Autodesk Inventor part; units mm, degrees
ref_plane "YZ Plane" through (0, 0, 0) normal (1, 0, 0) x (0, 1, 0)
ref_plane "XZ Plane" through (0, 0, 0) normal (0, 1, 0) x (-1, 0, 0)
ref_plane "XY Plane" through (0, 0, 0) normal (0, 0, 1) x (1, 0, 0)
sketch "Sketch1" plane through (0, 0, 0) normal (0, 0, 1) x (1, 0, 0)
  circle A0 centre (0, 0) radius 4
  dimension "Diameter" = 8
extrude "Extrusion1" add sketch "Sketch1" along normal blind 12
sketch "Sketch2" plane through (0, 0, 12) normal (0, 0, 1) x (1, 0, 0)
  circle A0 centre (0, 0) radius 4
  circle A1 centre (0, 0) radius 6.5
  dimension "Head_Diameter" = 13
extrude "Extrusion2" add sketch "Sketch2" along normal blind 8 contours A0 | A1
sketch "Sketch3" plane through (0, 0, 20) normal (0, 0, 1) x (1, 0, 0)
  circle A0 centre (0, 0) radius 6.5
  circle A1 centre (0, 0) radius 3.4641 construction
  line L0 (0, 3.4641) -> (3, 1.7321)
  line L1 (3, -1.7321) -> (3, 1.7321)
  line L2 (0, 3.4641) -> (-3, 1.7321)
  line L3 (-3, -1.7321) -> (-3, 1.7321)
  line L4 (-3, -1.7321) -> (0, -3.4641)
  line L5 (3, -1.7321) -> (0, -3.4641)
  dimension "Hex_Width" = 6
extrude "Extrusion3" cut sketch "Sketch3" against normal blind 4 contours L0 L1 L5 L4 L3 L2
thread "Thread1"
chamfer "Chamfer1" distance 0.8 angle 45 2 edges at (-6.5, 0, 20) (-4, 0, 0)
equation "\"d9\" = ThreadLength"
equation "\"d12\" = Chamfer"
equation "\"ThreadLength\" = 12"
properties part number "SCREW, SOCKET HD, P, 12.9, M8X1.25X12MM" material "Steel, MS"
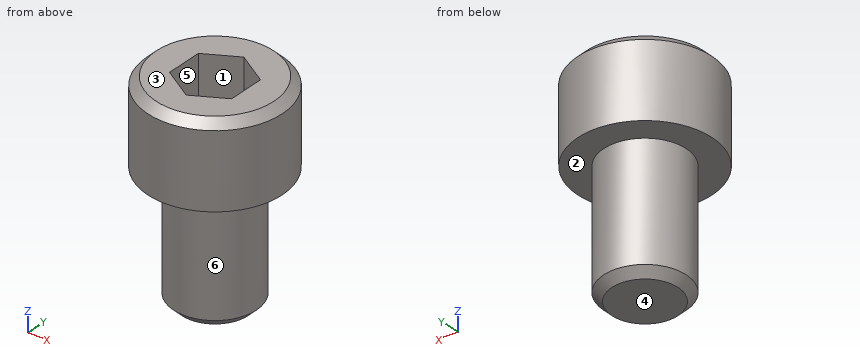
The model under review builds one solid part; all positions refer to its coordinate system, in mm. Face numbers are marked on the shaded views. A direction names the side the tool comes from. Coordinates: 2 decimals unless noted, no trailing zeros. Write each loop counter-clockwise with the first axis right and the second up, starting at its lowest first coordinate (ties: lowest second). Pieces come first, ordered by that corner, then holes. Notation, with made-up numbers: (-39.5, 57.25) - (-1.5, 57.25) arc R20 ccw to (-1.5, 83.25) - close; hole circle Ø6 at (-39, -12). An arc over 180 degrees is marked (long way). Answer as a JSON object with one key per item and string values. Group by question number.
1. To check wall thickness, follow probe 1 along Z at (x, y) = (0.5, -5); probe 2 along X at (y, z) = (-5.5, 17.75); probe 3 along Z at (x, y) = (-2, -0.75). State the ranges of each line that lie inside material, in increasing order.
2. Add section B-B (z = 15). Give the boundary of the cut face in (x, y).
3. Mouldability with a two-part tool opening along X and no side actions: class the marked faces 4, 5 and 6 as pulls with the +X half, pulls with the -X half, needs draft (parallel to the pull), parting line crosses it, or undercut.
4. Machinability: for the marked faces 1, 2 and 3, which of the approach directions +Z, -Z, +X, -X, +Y, -Y give a long, thin tool a straight path to every point of the face, cutting with its end or side? Answer none if there is none.
5. Add section C-C (z = 5.25). Give the boundary of the cut face in (x, y), plus the area to 3 significant figures.
6. Clearance check with flat-ended pins moving along their axes: pin 1 Ø3 at (x, y) = (-0.5, -5) entering from -Z; pin 2 Ø1.5 at (x, z) = (-2.5, 16.5) entering from +Y; pin 3 Ø1.8 at (x, y) = (-0.5, 0) entering from +Z. State where each tip first meets the part, or that it passes through.
7. Add section A-A (y = 0). Give the boundary of the cut face in (x, z), plus the area to 3 significant figures.
Findings:
{
 "1": {"probe 1": "12 to 20", "probe 2": "-3.46 to 3.46", "probe 3": "0 to 16"},
 "2": {"outline": "circle Ø13 at (0, 0)"},
 "3": {"face 4": "needs draft", "face 5": "undercut", "face 6": "parting line crosses it"},
 "4": {"face 1": "+Z", "face 2": "-Z", "face 3": "+Z, +X, -X, +Y, -Y"},
 "5": {"outline": "circle Ø8 at (0, 0)", "area": "50.3 mm²"},
 "6": {"pin 1": "z = 0.32", "pin 2": "y = 6.26", "pin 3": "z = 16"},
 "7": {"outline": "(-6.5, 12) - (-4, 12) - (-4, 0.8) - (-3.2, 0) - (3.2, 0) - (4, 0.8) - (4, 12) - (6.5, 12) - (6.5, 19.2) - (5.7, 20) - (3, 20) - (3, 16) - (-3, 16) - (-3, 20) - (-5.7, 20) - (-6.5, 19.2) - close", "area": "175 mm²"}
}
